```python
from build123d import *

# Parameters (mm, degrees)
F0_R     = 13.5
F1_DEPTH = 190
F0_R_2   = 25
F2_DEPTH = 5
F3_SIZE2 = 3.4641016151
F3_SIZE  = 2


with BuildPart() as f1:
    # F0 (on Right) → F1 (new body)
    with BuildSketch(Plane.YZ):
        Circle(F0_R)
    extrude(amount=F1_DEPTH)

    # F0 (on Right) → F2 (join)
    with BuildSketch(Plane.YZ):
        Circle(F0_R_2)
        Circle(F0_R, mode=Mode.SUBTRACT)
    extrude(amount=F2_DEPTH)

    # F3
    f3_edges = [f1.edges().sort_by_distance(p)[0] for p in [
        (190, -13.5, 0),
    ]]
    f3_side = f1.faces().sort_by_distance((190, 0, 0))[0]
    chamfer(f3_edges, length=F3_SIZE, length2=F3_SIZE2, reference=f3_side)


solid = f1.part
```
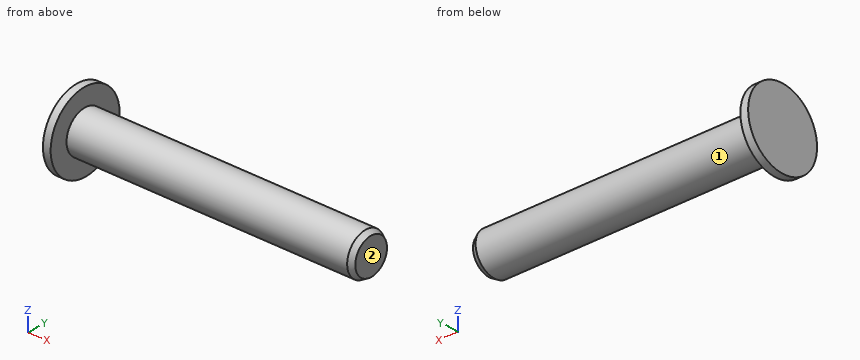
The model under review builds one solid part; all positions refer to its coordinate system, in mm. Face numbers are marked on the shaded views. A direction names the side the tool comes from. Give positions to 0.01 mm unless a question says otherwise; leave off trailing zeros. Write each loop counter-clockwise with the first axis right and the second up, starting at its lowest first coordinate (ties: lowest second). Pieces come first, ordered by that corner, then holes. Notation, with made-up numbers: (57, 29) -> (88, 29) arc R34 cw to (88, 62) -> close; hole circle Ø11 at (-24.5, -17.75). An arc over 180 degrees is marked (long way). Answer in a Markdown table with one row per item.
1) For L1, parallel to X at y = 17, z = -0.5; L2, parallel to Y at x = 11, z = 4; L3, parallel to Y at x = 87, z = -5, list the stretches that pass through material, from the lowest coordinate up. Write a range as [from, to].
Worked answers:
| item | result |
|---|---|
| L1 | [0, 5] |
| L2 | [-12.89, 12.89] |
| L3 | [-12.54, 12.54] |
2) Add section A-A on y = 0. State the section outline as (x, z) points, plus the area to 3 significant figures.
Worked answers:
| item | result |
|---|---|
| outline | (0, -25) -> (5, -25) -> (5, -13.5) -> (186.54, -13.5) -> (190, -11.5) -> (190, 11.5) -> (186.54, 13.5) -> (5, 13.5) -> (5, 25) -> (0, 25) -> close |
| area | 5,240 mm² |
3) Tool access review of the marked faces 1 and 2: name each direction out of +Z, -Z, +X, -X, +Y, -Y from which nothing blocks a thin tool from reaching the whole face with its end or side.
Worked answers:
| item | result |
|---|---|
| face 1 | +X |
| face 2 | +Z, -Z, +X, +Y, -Y |
4) Add section C-C on x = 87. State the section outline as (y, z) points, plus the area to 3 significant figures.
Worked answers:
| item | result |
|---|---|
| outline | circle Ø27 at (0, 0) |
| area | 573 mm² |
5) Add section D-D on y = -20. State the section outline as (x, z) points.
Worked answers:
| item | result |
|---|---|
| outline | (0, -15) -> (5, -15) -> (5, 15) -> (0, 15) -> close |
6) Clearance check with flat-ended pins moving along their axes: P1, Ø6, axis at x = 27.5, z = 6, coming from the +Y side; P2, Ø4, axis at x = 163.5, z = 6, coming from the -Y side; P3, Ø8, axis at x = 115, y = -11, coming from the -Z side. State where each tip first meets the part, or that it passes through.
Worked answers:
| item | result |
|---|---|
| P1 | y = 13.16 |
| P2 | y = -12.89 |
| P3 | z = -11.54 |
